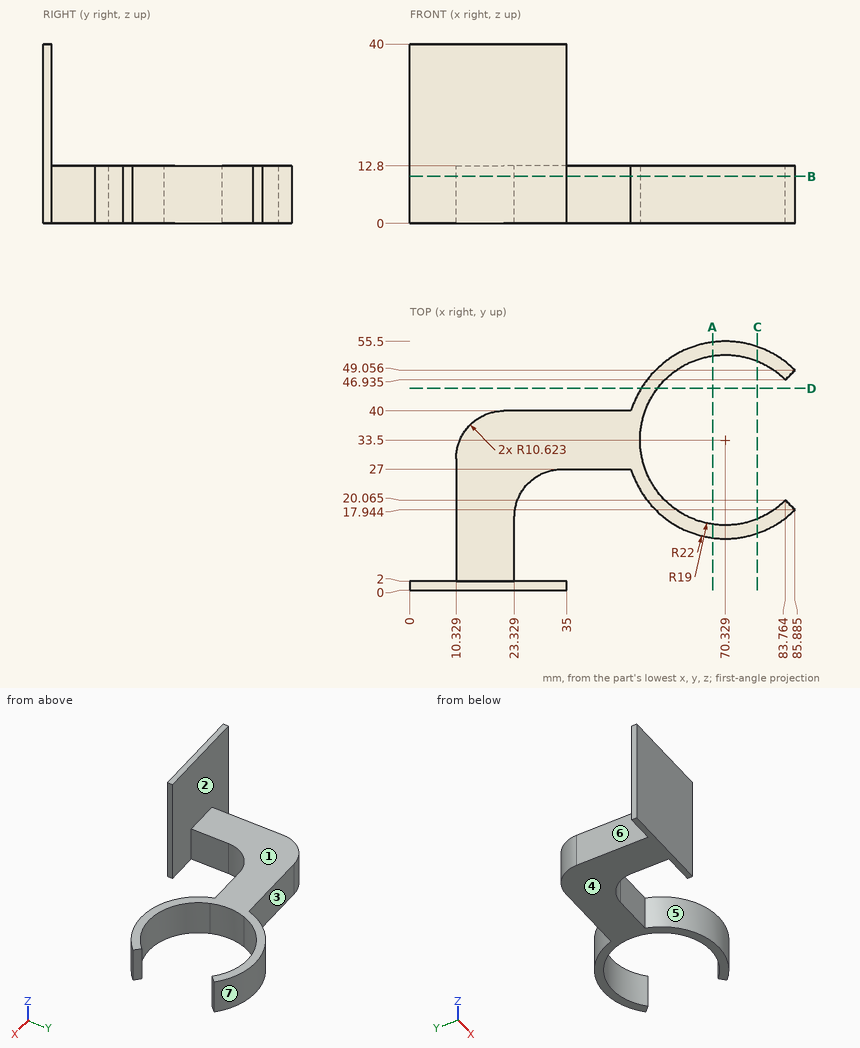
Geometry: see drawing. Coordinates: mm, zero at the bounding-box minimum. A direction names the side the tool comes from. Coordinates: 2 decimals unless noted, no trailing zeros. Loops run counter-clockwise (first coordinate to the right, second up) from the corner with the lowest first, then second, coordinate; pieces in that order, holes last. Notation, with made-up numbers: M 40.5,42.5 L 72.5,42.5 A21 cw 72.5,67.5 Z; hole C 6,1 d7. An arc over 180 degrees is marked long. Put each result on its own line as item: value. Start each with the question number.
1) Cut plane B-B on z = 10.5. Return the cut outline in (x, y) (1 decimal).
2) Pull-direction query (X, two-part tool) for the marked faces 4, 5, 6 and 7; classes: pulls with the +X half, pulls with the -X half, needs draft (parallel to the pull), parting line crosses it, or undercut.
3) Reachability of the marked faces 1, 2 and 3 from +Z, -Z, +X, -X, +Y, -Y: full face, straight path, thin tool, end or side. Return the list, or none.
4) Cut plane A-A on x = 67.5. Return the cut outline in (y, z).
5) Cut plane C-C on x = 77.5. Return the cut outline in (y, z) (1 decimal).
6) Contact query for flat-ended pins moving along their axis: pin 1 Ø0.6 at (y, z) = (0.5, 14.5) entering from +X; pin 2 Ø10 at (x, z) = (40.5, 5.5) entering from +Y; pin 3 Ø12 at (y, z) = (13.5, 5) entering from +X (1 decimal). Output: stop coordinate, or through.
7) Ray query, L1, parallel to Y at x = 4.5, z = 2; L2, parallel to Z at x = 44, y = 35; L3, parallel to X at y = 5.5, z = 5.5. Return the intervals inside material, ascending. Write a range as from..to.
8) Cut plane D-D on y = 45. Return the cut outline in (x, z) (1 decimal).
The answers:
1. outline: M 0,0 L 35,0 L 35,2 L 23.3,2 L 23.3,16.4 A10.6 cw 34,27 L 49.3,27 A22 ccw 85.9,17.9 L 83.8,20.1 A19 cw long 83.8,46.9 L 85.9,49.1 A22 ccw 49.3,40 L 21,40 A10.6 ccw 10.3,29.4 L 10.3,2 L 0,2 Z
2. face 4: needs draft
2. face 5: undercut
2. face 6: pulls with the -X half
2. face 7: parting line crosses it
3. face 1: +Z, +X, -X, +Y
3. face 2: +Z
3. face 3: +Z, -Z, -X, +Y
4. outline: M 11.68,0 L 14.71,0 L 14.71,12.8 L 11.68,12.8 Z; M 52.29,0 L 55.32,0 L 55.32,12.8 L 52.29,12.8 Z
5. outline: M 12.7,0 L 15.9,0 L 15.9,12.8 L 12.7,12.8 Z; M 51.1,0 L 54.3,0 L 54.3,12.8 L 51.1,12.8 Z
6. pin 1: stops at x = 35
6. pin 2: stops at y = 40
6. pin 3: stops at x = 85.9
7. L1: y = 0..2
7. L2: z = 0..12.8
7. L3: x = 10.33..23.33
8. outline: M 51.6,0 L 55.2,0 L 55.2,12.8 L 51.6,12.8 Z
